Geometry check sheet. Reference: the model listing, model coordinates, mm. Face numbers are marked on the shaded views. A direction names the side the tool comes from. Round coordinates to 2 decimals unless told otherwise and drop trailing zeros. Loops run counter-clockwise (first coordinate to the right, second up) from the corner with the lowest first, then second, coordinate; pieces in that order, holes last. Notation, with made-up numbers: M -38,-23 L -5,-23 A8 ccw -5,-13 Z; hole C -29.75,12.25 d6. An arc over 180 degrees is marked long. Answer in a Markdown table with one row per item. Add a question column.
```python
from build123d import *

# Parameters (mm, degrees)
SKETCH1_W          = 20.701
SKETCH1_H          = 6.223
EXTRUDE1_DEPTH     = 8.636
CUT_EXTRUDE1_DEPTH = 25.4
CUT_EXTRUDE2_DEPTH = 25.4
SKETCH4_R          = 1.016
CUT_EXTRUDE3_DEPTH = 0.508
CUT_EXTRUDE4_DEPTH = 0.508
SKETCH6_W          = 1.82195604
SKETCH6_H          = 3.576432228
CUT_EXTRUDE5_DEPTH = 1.27
CHAMFER1_SIZE      = 0.508
SKETCH7_W          = 0.80595604
SKETCH7_H          = 0.757943843
CUT_EXTRUDE6_DEPTH = 1.27
SKETCH8_W          = 0.433382436
SKETCH8_H          = 0.491166761
EXTRUDE2_DEPTH     = 1.905
SKETCH9_W          = 13.835725518
SKETCH9_H          = 11.068580414
CUT_EXTRUDE7_DEPTH = 25.4


with BuildPart() as part:
    # Sketch1 → Extrude1 (new body)
    with BuildSketch(Plane(origin=(0, 0, 0), x_dir=(1, 0, 0), z_dir=(0, 1, 0))):
        with Locations((10.3505, 3.1115)):
            Rectangle(SKETCH1_W, SKETCH1_H)
    extrude(amount=EXTRUDE1_DEPTH)

    # Sketch2 → Cut-Extrude1 (cut)
    with BuildSketch(Plane(origin=(20.701, 0, 0), x_dir=(0, 0, -1), z_dir=(1, 0, 0))):
        Polygon((-2.869110069, 4.645946632), (0.62179162, 4.645946632), (2.217632392, 11.827230107), (-2.869110069, 11.827230107), align=None)
    extrude(amount=-CUT_EXTRUDE1_DEPTH, mode=Mode.SUBTRACT)

    # Sketch3 → Cut-Extrude2 (cut)
    with BuildSketch(Plane(origin=(20.701, 0, 0), x_dir=(0, 0, -1), z_dir=(1, 0, 0))):
        Polygon((4.012953261, 10.231389335), (6.905414661, 0.855824797), (9.199435771, 0.855824797), (9.199435771, 10.231389335), align=None)
    extrude(amount=-CUT_EXTRUDE2_DEPTH, mode=Mode.SUBTRACT)

    # Sketch4 → Cut-Extrude3 (cut)
    with BuildSketch(Plane(origin=(0, 8.636, 0), x_dir=(1, 0, 0), z_dir=(0, 1, 0))):
        with Locations(Location((1.27, 2.949100672, 0), (0, 0, 270))):
            Circle(SKETCH4_R)
        with Locations(Location((3.81, 2.949100672, 0), (0, 0, 270))):
            Circle(SKETCH4_R)
        with Locations(Location((6.35, 2.949100672, 0), (0, 0, 270))):
            Circle(SKETCH4_R)
        with Locations(Location((8.89, 2.949100672, 0), (0, 0, 270))):
            Circle(SKETCH4_R)
        with Locations(Location((11.43, 2.949100672, 0), (0, 0, 270))):
            Circle(SKETCH4_R)
        with Locations(Location((13.97, 2.949100672, 0), (0, 0, 270))):
            Circle(SKETCH4_R)
        with Locations(Location((16.51, 2.949100672, 0), (0, 0, 270))):
            Circle(SKETCH4_R)
        with Locations(Location((19.05, 2.949100672, 0), (0, 0, 270))):
            Circle(SKETCH4_R)
    extrude(amount=-CUT_EXTRUDE3_DEPTH, mode=Mode.SUBTRACT)

    # Sketch5 → Cut-Extrude4 (cut)
    with BuildSketch(Plane(origin=(0, 8.128, 0), x_dir=(1, 0, 0), z_dir=(0, 1, 0))):
        with BuildLine():
            ThreePointArc((0.55685802, 3.67276117), (0.471993814, 3.577942566), (0.399647546, 3.473259623))
            Line((0.399647546, 3.473259623), (1.98314198, 2.225440174))
            ThreePointArc((1.98314198, 2.225440174), (2.068006186, 2.320258778), (2.140352454, 2.42494172))
            Line((2.140352454, 2.42494172), (0.55685802, 3.67276117))
        make_face()
        with BuildLine():
            ThreePointArc((2.939647546, 2.42494172), (3.011993814, 2.320258778), (3.09685802, 2.225440174))
            Line((3.09685802, 2.225440174), (4.680352454, 3.473259623))
            ThreePointArc((4.680352454, 3.473259623), (4.608006186, 3.577942566), (4.52314198, 3.67276117))
            Line((4.52314198, 3.67276117), (2.939647546, 2.42494172))
        make_face()
        with BuildLine():
            ThreePointArc((5.34196875, 3.076100672), (5.334, 2.949100672), (5.34196875, 2.822100672))
            Line((5.34196875, 2.822100672), (7.35803125, 2.822100672))
            ThreePointArc((7.35803125, 2.822100672), (7.364005855, 2.885475793), (7.366, 2.949100672))
            ThreePointArc((7.366, 2.949100672), (7.364005855, 3.012725551), (7.35803125, 3.076100672))
            Line((7.35803125, 3.076100672), (5.34196875, 3.076100672))
        make_face()
        with BuildLine():
            ThreePointArc((8.458529789, 2.041483422), (8.576688012, 1.994233554), (8.699870069, 1.9622946))
            Line((8.699870069, 1.9622946), (9.321470211, 3.856717921))
            ThreePointArc((9.321470211, 3.856717921), (9.203311988, 3.90396779), (9.080129931, 3.935906744))
            Line((9.080129931, 3.935906744), (8.458529789, 2.041483422))
        make_face()
        with BuildLine():
            ThreePointArc((11.557, 3.957131921), (11.43, 3.965100672), (11.303, 3.957131921))
            Line((11.303, 3.957131921), (11.303, 1.941069422))
            ThreePointArc((11.303, 1.941069422), (11.43, 1.933100672), (11.557, 1.941069422))
            Line((11.557, 1.941069422), (11.557, 3.957131921))
        make_face()
        with BuildLine():
            ThreePointArc((13.060727808, 3.402399778), (13.011197076, 3.285185412), (12.976706622, 3.162699047))
            Line((12.976706622, 3.162699047), (14.879272192, 2.495801565))
            ThreePointArc((14.879272192, 2.495801565), (14.928802924, 2.613015931), (14.963293378, 2.735502296))
            Line((14.963293378, 2.735502296), (13.060727808, 3.402399778))
        make_face()
        with BuildLine():
            ThreePointArc((16.944941036, 3.867295801), (16.826755289, 3.914461789), (16.703600756, 3.946484624))
            Line((16.703600756, 3.946484624), (16.075058964, 2.030905542))
            ThreePointArc((16.075058964, 2.030905542), (16.193244711, 1.983739555), (16.316399244, 1.95171672))
            Line((16.316399244, 1.95171672), (16.944941036, 3.867295801))
        make_face()
        with BuildLine():
            ThreePointArc((18.349819557, 3.662547267), (18.264852019, 3.567810091), (18.192609083, 3.463045721))
            Line((18.192609083, 3.463045721), (19.750180443, 2.235654077))
            ThreePointArc((19.750180443, 2.235654077), (19.835147981, 2.330391253), (19.907390917, 2.435155623))
            Line((19.907390917, 2.435155623), (18.349819557, 3.662547267))
        make_face()
    extrude(amount=-CUT_EXTRUDE4_DEPTH, mode=Mode.SUBTRACT)

    # Sketch6 → Cut-Extrude5 (cut)
    with BuildSketch(Plane.XY):
        with Locations((3.861070401, 2.24061075)):
            Rectangle(SKETCH6_W, SKETCH6_H)
        with Locations((1.321070401, 2.24061075)):
            Rectangle(SKETCH6_W, SKETCH6_H)
        with Locations((6.401070401, 2.24061075)):
            Rectangle(SKETCH6_W, SKETCH6_H)
        with Locations((8.941070401, 2.24061075)):
            Rectangle(SKETCH6_W, SKETCH6_H)
        with Locations((11.481070401, 2.24061075)):
            Rectangle(SKETCH6_W, SKETCH6_H)
        with Locations((14.021070401, 2.24061075)):
            Rectangle(SKETCH6_W, SKETCH6_H)
        with Locations((16.561070401, 2.24061075)):
            Rectangle(SKETCH6_W, SKETCH6_H)
        with Locations((19.101070401, 2.24061075)):
            Rectangle(SKETCH6_W, SKETCH6_H)
    extrude(amount=-CUT_EXTRUDE5_DEPTH, mode=Mode.SUBTRACT)

    # Chamfer1
    chamfer1_edges = [part.edges().sort_by_distance(p)[0] for p in [
        (0.410092381, 2.24061075, -1.27),
        (1.321070401, 4.028826864, -1.27),
        (2.232048421, 2.24061075, -1.27),
        (1.321070401, 0.452394636, -1.27),
        (3.861070401, 4.028826864, -1.27),
        (4.772048421, 2.24061075, -1.27),
        (3.861070401, 0.452394636, -1.27),
        (2.950092381, 2.24061075, -1.27),
        (6.401070401, 4.028826864, -1.27),
        (7.312048421, 2.24061075, -1.27),
        (6.401070401, 0.452394636, -1.27),
        (5.490092381, 2.24061075, -1.27),
        (8.941070401, 4.028826864, -1.27),
        (9.852048421, 2.24061075, -1.27),
        (8.941070401, 0.452394636, -1.27),
        (8.030092381, 2.24061075, -1.27),
        (11.481070401, 4.028826864, -1.27),
        (12.392048421, 2.24061075, -1.27),
        (11.481070401, 0.452394636, -1.27),
        (10.570092381, 2.24061075, -1.27),
        (14.021070401, 4.028826864, -1.27),
        (14.932048421, 2.24061075, -1.27),
        (14.021070401, 0.452394636, -1.27),
        (13.110092381, 2.24061075, -1.27),
        (16.561070401, 4.028826864, -1.27),
        (17.472048421, 2.24061075, -1.27),
        (16.561070401, 0.452394636, -1.27),
        (15.650092381, 2.24061075, -1.27),
        (19.101070401, 4.028826864, -1.27),
        (20.012048421, 2.24061075, -1.27),
        (19.101070401, 0.452394636, -1.27),
        (18.190092381, 2.24061075, -1.27),
    ]]
    chamfer(chamfer1_edges, length=CHAMFER1_SIZE)

    # Sketch7 → Cut-Extrude6 (cut)
    with BuildSketch(Plane.XY.offset(-1.27)):
        with Locations((1.321070401, 2.17271271)):
            Rectangle(SKETCH7_W, SKETCH7_H)
        with Locations((3.861070401, 2.17271271)):
            Rectangle(SKETCH7_W, SKETCH7_H)
        with Locations((6.401070401, 2.17271271)):
            Rectangle(SKETCH7_W, SKETCH7_H)
        with Locations((8.941070401, 2.17271271)):
            Rectangle(SKETCH7_W, SKETCH7_H)
        with Locations((11.481070401, 2.17271271)):
            Rectangle(SKETCH7_W, SKETCH7_H)
        with Locations((14.021070401, 2.17271271)):
            Rectangle(SKETCH7_W, SKETCH7_H)
        with Locations((16.561070401, 2.17271271)):
            Rectangle(SKETCH7_W, SKETCH7_H)
        with Locations((19.101070401, 2.17271271)):
            Rectangle(SKETCH7_W, SKETCH7_H)
    extrude(amount=-CUT_EXTRUDE6_DEPTH, mode=Mode.SUBTRACT)

    # Sketch8 → Extrude2 (add)
    with BuildSketch(Plane.XZ):
        with Locations((3.829530977, -2.990246105)):
            Rectangle(SKETCH8_W, SKETCH8_H)
        with Locations((1.289530977, -2.990246105)):
            Rectangle(SKETCH8_W, SKETCH8_H)
        with Locations((6.369530977, -2.990246105)):
            Rectangle(SKETCH8_W, SKETCH8_H)
        with Locations((8.909530977, -2.990246105)):
            Rectangle(SKETCH8_W, SKETCH8_H)
        with Locations((11.449530977, -2.990246105)):
            Rectangle(SKETCH8_W, SKETCH8_H)
        with Locations((13.989530977, -2.990246105)):
            Rectangle(SKETCH8_W, SKETCH8_H)
        with Locations((16.529530977, -2.990246105)):
            Rectangle(SKETCH8_W, SKETCH8_H)
        with Locations((19.069530977, -2.990246105)):
            Rectangle(SKETCH8_W, SKETCH8_H)
    extrude(amount=EXTRUDE2_DEPTH)

    # Sketch9 → Cut-Extrude7 (cut)
    with BuildSketch(Plane(origin=(0, 8.636, 0), x_dir=(1, 0, 0), z_dir=(0, 1, 0))):
        with Locations((14.474610491, 2.472928053)):
            Rectangle(SKETCH9_W, SKETCH9_H)
    extrude(amount=-CUT_EXTRUDE7_DEPTH, mode=Mode.SUBTRACT)


solid = part.part
```
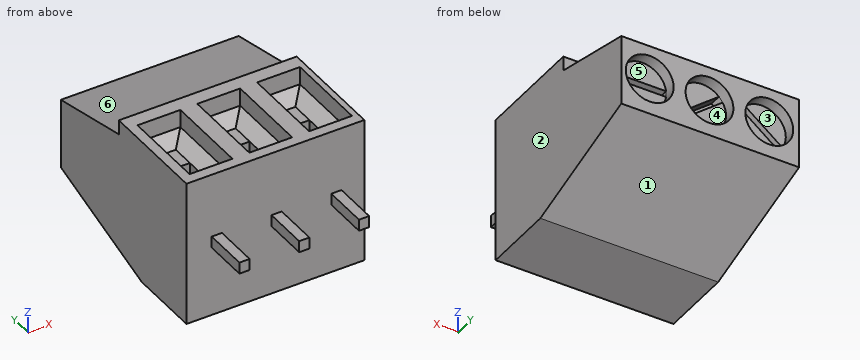
1) Cross-section at D-D, the plane z = -5.5. Record the boundary of the cut face in (x, y).
2) Draft check along Z on the marked faces 1, 2, 3 and 4. Enter one of: +Z half, -Z half, draft (parallel to the pull), parting line (faces both ways), or undercut.
3) Cross-section at C-C, the plane y = 2.75. Record the boundary of the cut face in (x, z), plus the area to 3 significant figures.
4) Thickness scan on L1, parallel to Y at x = 6, z = -0.5; L2, parallel to Z at x = 6.5, y = 1; L3, parallel to Y at x = 4.5, z = -3. Record the ranges inside material, lowest first. Write a range as [from, to].
5) Go/stop test with flat-tipped pins: pin 1 (0.6 mm diameter, centred on x = 4, y = 3, fed in from +Z); pin 2 (0.8 mm diameter, centred on x = 1, z = -0.5, fed in from -Y). Record where each tip stops, or that it passes through.
6) Set-up check for the marked faces 5 and 6: record each of +Z, -Z, +X, -X, +Y, -Y from which the full face is reachable in a straight line by a thin tool's end or side.
7) Cross-section at A-A, the plane z = -1.75. Record the boundary of the cut face in (x, y).
Worked answers:
| question | item | result |
|---|---|---|
| 1 | outline | M 0,0 L 7.56,0 L 7.56,5.41 L 0,5.41 Z |
| 2 | face 1 | -Z half |
| 2 | face 2 | draft |
| 2 | face 3 | undercut |
| 2 | face 4 | undercut |
| 3 | outline | M 0,-6.22 L 7.56,-6.22 L 7.56,0 L 7.31,0 L 7.31,-0.76 L 6.8,-1.27 L 6,-1.27 L 5.49,-0.76 L 5.49,0 L 4.77,0 L 4.77,-0.76 L 4.26,-1.27 L 3.46,-1.27 L 2.95,-0.76 L 2.95,0 L 2.23,0 L 2.23,-0.76 L 1.72,-1.27 L 0.92,-1.27 L 0.41,-0.76 L 0.41,0 L 0,0 Z |
| 3 | area | 40.9 mm2 |
| 4 | L1 | y = [0, 0.45], [4.03, 4.65] |
| 4 | L2 | z = [-6.22, -1.27] |
| 4 | L3 | y = [0, 8.13] |
| 5 | pin 1 | stops at z = -1.23 |
| 5 | pin 2 | stops at y = 0 |
| 6 | face 5 | +Y |
| 6 | face 6 | +Z, +X, -X, +Y |
| 7 | outline | M 0,0 L 7.56,0 L 7.56,8.64 L 0,8.64 Z; hole M 0.92,1.79 L 1.72,1.79 L 1.72,2.55 L 0.92,2.55 Z; hole M 3.46,1.79 L 4.26,1.79 L 4.26,2.55 L 3.46,2.55 Z; hole M 6,1.79 L 6.8,1.79 L 6.8,2.55 L 6,2.55 Z |
